Autodesk Inventor part; units mm, degrees
ref_plane "YZ Plane" through (0, 0, 0) normal (1, 0, 0) x (0, 1, 0)
ref_plane "XZ Plane" through (0, 0, 0) normal (0, 1, 0) x (-1, 0, 0)
ref_plane "XY Plane" through (0, 0, 0) normal (0, 0, 1) x (1, 0, 0)
sketch "スケッチ1" plane through (0, 0, 0) normal (0, 1, 0) x (-1, 0, 0)
  line L0 (-42, -25) -> (42, -25)
  line L1 (42, -25) -> (42, 25)
  line L2 (42, 25) -> (-42, 25)
  line L3 (-42, 25) -> (-42, -25)
  line L4 (-42, -25) -> (42, 25) construction
  line L5 (42, -25) -> (-42, 25) construction
  point P0 (0, 0)
  dimension "d0" = 84
  dimension "d1" = 50
extrude "プレート1" add sketch "スケッチ1" along normal blind 2
sketch "スケッチ2" plane through (-42, 0, -25) normal (-1, 0, 0) x (0, 0, 1)
  line L0 (0, 0) -> (50, 0)
  line L1 (50, 0) -> (0, 0)
  line L2 (0, 0) -> (0, 20)
  line L3 (0, 20) -> (50, 20)
  line L4 (50, 20) -> (50, 0)
  point P0 (25, 0)
  dimension "d3" = 20
sheet face with bend "面2" sketch "スケッチ2" thickness 2 toward (1, 0, 0) bend radius 2
bend "曲げ1"
sketch "スケッチ3" plane through (42, 0, 25) normal (1, 0, 0) x (0, 0, -1)
  line L0 (0, 0) -> (50, 0)
  line L1 (50, 0) -> (50, 20)
  line L2 (50, 20) -> (0, 20)
  line L3 (0, 20) -> (0, 0)
  point P0 (25, 0)
  point P1 (50, 0)
  dimension "d9" = 20
sheet face with bend "面3" sketch "スケッチ3" thickness 2 toward (-1, 0, 0) bend radius 2
bend "曲げ2"
sketch "スケッチ4" plane through (0, 2, 0) normal (0, 1, 0) x (1, 0, 0)
  line L0 (-32, -15) -> (32, -15)
  arc A0 (32, -15) -> (32, -11) centre (32, -13) ccw
  line L1 (32, -11) -> (-32, -11)
  arc A1 (-32, -11) -> (-32, -15) centre (-32, -13) ccw
  line L2 (-18, -5) -> (18, -5)
  arc A2 (18, -5) -> (18, 5) centre (18, 0) ccw
  line L3 (18, 5) -> (-18, 5)
  arc A3 (-18, 5) -> (-18, -5) centre (-18, 0) ccw
  line L4 (-32, 11) -> (32, 11)
  arc A4 (32, 11) -> (32, 15) centre (32, 13) ccw
  line L5 (32, 15) -> (-32, 15)
  arc A5 (-32, 15) -> (-32, 11) centre (-32, 13) ccw
  line L6 (38, -25) -> (-38, -25)
  line L7 (38, -25) -> (38, 25)
  line L8 (-38, 25) -> (-38, -25)
  line L9 (-38, 25) -> (38, 25)
  point P0 (0, 0)
  dimension "d15" = 2
  dimension "d16" = 2
  dimension "d17" = 12
  dimension "d18" = 6
  dimension "d19" = 6
  dimension "d20" = 6
  dimension "d21" = 6
  dimension "d22" = 12
  dimension "d23" = 20
  dimension "d24" = 20
  dimension "d25" = 10
extrude "押し出し1" cut sketch "スケッチ4" against normal blind 10 contours A1 L1 A0 L0 | A3 L3 A2 L2 | A5 L5 A4 L4
sketch "スケッチ5" plane through (-42, 0, -25) normal (-1, 0, 0) x (0, 0, 1)
  line L0 (3, 16) -> (3, 8)
  arc A0 (3, 8) -> (7, 8) centre (5, 8) ccw
  line L1 (7, 8) -> (7, 16)
  arc A1 (7, 16) -> (3, 16) centre (5, 16) ccw
  line L2 (43, 16) -> (43, 8)
  arc A2 (43, 8) -> (47, 8) centre (45, 8) ccw
  line L3 (47, 8) -> (47, 16)
  arc A3 (47, 16) -> (43, 16) centre (45, 16) ccw
  line L4 (50, 4) -> (50, 20)
  line L5 (0, 20) -> (0, 4)
  line L6 (50, 20) -> (0, 20)
  line L7 (50, 4) -> (0, 4)
  point P0 (25, 0)
  dimension "d28" = 2
  dimension "d29" = 2
  dimension "d30" = 5
  dimension "d31" = 5
  dimension "d32" = 4
  dimension "d33" = 4
  dimension "d34" = 4
  dimension "d35" = 4
extrude "押し出し2" cut sketch "スケッチ5" against normal blind 10 contours A1 L1 A0 L0 | A3 L3 A2 L2
sketch "スケッチ6" plane through (42, 0, 25) normal (1, 0, 0) x (0, 0, -1)
  line L0 (13, 16) -> (13, 8)
  arc A0 (13, 8) -> (17, 8) centre (15, 8) ccw
  line L1 (17, 8) -> (17, 16)
  arc A1 (17, 16) -> (13, 16) centre (15, 16) ccw
  line L2 (33, 16) -> (33, 8)
  arc A2 (33, 8) -> (37, 8) centre (35, 8) ccw
  line L3 (37, 8) -> (37, 16)
  arc A3 (37, 16) -> (33, 16) centre (35, 16) ccw
  line L4 (50, 4) -> (50, 20)
  line L5 (0, 20) -> (0, 4)
  line L6 (50, 20) -> (0, 20)
  line L7 (50, 4) -> (0, 4)
  point P0 (25, 0)
  dimension "d38" = 2
  dimension "d39" = 2
  dimension "d40" = 15
  dimension "d41" = 15
  dimension "d42" = 4
  dimension "d43" = 4
extrude "押し出し3" cut sketch "スケッチ6" against normal blind 10 contours A1 L1 A0 L0 | A3 L3 A2 L2
equation "\"d2\" = Thickness"
equation "\"d4\" = BendRadius"
equation "\"d5\" = BendReliefWidth"
equation "\"d7\" = MinimumRemnant"
equation "\"d6\" = BendReliefDepth"
equation "\"d8\" = TransitionRadius"
equation "\"d10\" = BendRadius"
equation "\"d11\" = BendReliefWidth"
equation "\"d13\" = MinimumRemnant"
equation "\"d12\" = BendReliefDepth"
equation "\"d14\" = TransitionRadius"
equation "\"BendRadius\" = Thickness"
equation "\"BendReliefWidth\" = Thickness"
equation "\"BendReliefDepth\" = 0.5 * Thickness"
equation "\"CornerReliefSize\" = 4 * Thickness"
equation "\"MinimumRemnant\" = 2 * Thickness"
equation "\"TransitionRadius\" = BendRadius"
equation "\"JacobiRadiusSize\" = BendRadius"
equation "\"GapSize\" = Thickness"
properties part number "palmrest_cup" material "アルミニウム 6061"
Check sheet for the modelled part. Datum: model origin and axes. Units: mm. A direction names the side the tool comes from. Round coordinates to 2 decimals unless told otherwise and drop trailing zeros. Order: outer loops, then holes, each group sorted by start corner. A loop starts at its lowest first (then second) coordinate and runs counter-clockwise, first axis right, second up. Notation, with made-up numbers: (-28.75, 12.5) - (27.25, 12.5) arc R23 ccw to (27.25, 34.5) - close; hole circle Ø9 at (73.25, 5). An arc over 180 degrees is marked (long way). Answer as CSV lines item,"result". Start each with the question number.
1) Scan lines: probe 1 along X at (y, z) = (9.25, 3); probe 2 along Y at (x, z) = (32.5, -5.5); probe 3 along X at (y, z) = (3, -19). Record each from-to range of solid material in increasing order.
2) Section check B-B (y = 10.25). Record the cut outline in (x, z).
3) Section check A-A (z = -4). Record the cut outline in (x, y).
4) Section check D-D (z = 17). Record the cut outline in (x, y), then the cut area to 3 significant figures.
5) Section check C-C (x = 0). Record the cut outline in (y, z).
6) Draft check along Z on faces 5 (the face through (34, 1, -13)), 6 (the face through (40.859, 1.203, -0.35)). Enter one of: +Z half, -Z half, draft (parallel to the pull), parting line (faces both ways), or undercut.
7) Tool access check on faces 1 (the face through (0.5, 0, -5.2)), 2 (the face through (41, 6, 10)), 3 (the face through (-41, 6, 20)), 4 (the face through (-23, 1, 0)). Record the directions out of +Z, -Z, +X, -X, +Y, -Y that give a thin tool (end or side, any length) a straight path to the whole face; none if there is none.
8) Depth check by flat-ended pin: pin 1 (10 mm diameter, centred on x = -29, z = -11, fed in from +Y). Enter the tip coordinate at first touch or a pass-through.
Determined:
1,probe 1,"-42 to -40, 40 to 42"
1,probe 2,"0 to 2"
1,probe 3,"-41.87 to -39.73, 39.73 to 41.87"
2,outline,"(-42, -25) - (-40, -25) - (-40, -22) - (-42, -22) - close; (-42, -18) - (-40, -18) - (-40, 18) - (-42, 18) - close; (-42, 22) - (-40, 22) - (-40, 25) - (-42, 25) - close; (40, -25) - (42, -25) - (42, -12) - (40, -12) - close; (40, -8) - (42, -8) - (42, 8) - (40, 8) - close; (40, 12) - (42, 12) - (42, 25) - (40, 25) - close"
3,outline,"(-42, 4) arc R4 ccw to (-38, 0) - (-21, 0) - (-21, 2) - (-38, 2) arc R2 cw to (-40, 4) - (-40, 20) - (-42, 20) - close; (21, 0) - (38, 0) arc R4 ccw to (42, 4) - (42, 20) - (40, 20) - (40, 4) arc R2 cw to (38, 2) - (21, 2) - close"
4,outline,"(-42, 4) arc R4 ccw to (-38, 0) - (38, 0) arc R4 ccw to (42, 4) - (42, 20) - (40, 20) - (40, 4) arc R2 cw to (38, 2) - (-38, 2) arc R2 cw to (-40, 4) - (-40, 20) - (-42, 20) - close"
4,area,"235 mm^2"
5,outline,"(0, -25) - (2, -25) - (2, -15) - (0, -15) - close; (0, -11) - (2, -11) - (2, -5) - (0, -5) - close; (0, 5) - (2, 5) - (2, 11) - (0, 11) - close; (0, 15) - (2, 15) - (2, 25) - (0, 25) - close"
6,face 5,"undercut"
6,face 6,"draft"
7,face 1,"+Z, -Z, +X, -X, -Y"
7,face 2,"+X"
7,face 3,"-X"
7,face 4,"+Y, -Y"
8,pin 1,"y = 2"
